For this review, take the finished solid that the model builds, in its own axes (mm). A direction names the side the tool comes from. Give positions to 0.01 mm unless a question says otherwise; leave off trailing zeros. Order: outer loops, then holes, each group sorted by start corner. A loop starts at its lowest first (then second) coordinate and runs counter-clockwise, first axis right, second up.
Item 1: Consider section A-A (x = -25.5). Give the boundary of the cut face in (y, z), plus the area to 3 significant figures.
Item 2: The part is to be moulded in two halves that separate along X. For faces 1 (the flat face through (-19.231, -31.307, 8.381)), 2 (the flat face through (-25, -21.047, 5)), 3 (the flat face through (-29.73, -31.34, 8.38)), 4 (the flat face through (-19.472, -26, 5)), say which applies: released by +X, released by -X, zero draft, split by the parting line, or undercut.
Item 3: Consider section C-C (z = 9.75). Give the boundary of the cut face in (x, y), plus the area to 3 significant figures.
Item 4: Consider section B-B (z = 15.25). Give the boundary of the cut face in (x, y), plus the area to 3 significant figures.
Item 5: For probe 1 along Y at (x, z) = (-25.5, 10); probe 2 along X at (y, z) = (-28, 1.75); probe 3 along Z at (x, y) = (-21.5, -30.25), list the stretches that pass through material, from the lowest coordinate up.
Item 6: Machinability: for faces 5 (the flat face through (-29.522, -26, 5)), 6 (the flat face through (-30.847, -26, 8)), which of the approach directions +Z, -Z, +X, -X, +Y, -Y give a long, thin tool a straight path to every point of the face, cutting with its end or side? Answer none if there is none.
```python
from build123d import *

# Parameters (mm, degrees)
F0_W     = 12.7
F0_H     = 12.7
F0_W_2   = 10.05
F0_H_2   = 10.05
F1_DEPTH = 17
F2_DEPTH = 17
F3_DEPTH = 11
F4_SIZE  = 2.2
F5_R     = 1.9


with BuildPart() as f1:
    # F0 (on Top) → F1 (new body)
    with BuildSketch(Plane.XY):
        with Locations((-24.496685, -26.072449)):
            Rectangle(F0_W, F0_H)
        with Locations((-24.496685, -26.072449)):
            Rectangle(F0_W_2, F0_H_2, mode=Mode.SUBTRACT)
    extrude(amount=F1_DEPTH)

    # F0 (on Top) → F2 (join)
    with BuildSketch(Plane.XY):
        with Locations((-24.496685, -26.072449)):
            Rectangle(F0_W_2, F0_H_2)
    extrude(amount=F2_DEPTH)

    # F0 (on Top) → F3 (cut)
    with BuildSketch(Plane.XY):
        with Locations((-24.496685, -26.072449)):
            Rectangle(F0_W_2, F0_H_2)
    extrude(amount=F3_DEPTH, mode=Mode.SUBTRACT)

    # F4
    f4_edges = [f1.edges().sort_by_distance(p)[0] for p in [
        (-18.146685, -19.722449, 8.5),
        (-30.846685, -19.722449, 8.5),
        (-30.846685, -32.422449, 8.5),
        (-18.146685, -32.422449, 8.5),
    ]]
    chamfer(f4_edges, length=F4_SIZE)

    # F5
    f5_edges = [f1.edges().sort_by_distance(p)[0] for p in [
        (-19.471685, -31.097449, 5.5),
        (-19.471685, -21.047449, 5.5),
        (-29.521685, -21.047449, 5.5),
        (-29.521685, -31.097449, 5.5),
    ]]
    fillet(f5_edges, radius=F5_R)


solid = f1.part
```
Resolved:
1. outline: (-32.42, 0) - (-31.1, 0) - (-31.1, 11) - (-21.05, 11) - (-21.05, 0) - (-19.72, 0) - (-19.72, 17) - (-32.42, 17) - close
1. area: 105 mm2
2. face 1: released by +X
2. face 2: undercut
2. face 3: released by -X
2. face 4: undercut
3. outline: (-30.85, -30.22) - (-28.65, -32.42) - (-20.35, -32.42) - (-18.15, -30.22) - (-18.15, -21.92) - (-20.35, -19.72) - (-28.65, -19.72) - (-30.85, -21.92) - close; hole (-29.52, -29.2) arc R1.9 ccw to (-27.62, -31.1) - (-21.37, -31.1) arc R1.9 ccw to (-19.47, -29.2) - (-19.47, -22.95) arc R1.9 ccw to (-21.37, -21.05) - (-27.62, -21.05) arc R1.9 ccw to (-29.52, -22.95) - close
3. area: 53.7 mm2
4. outline: (-30.85, -30.22) - (-28.65, -32.42) - (-20.35, -32.42) - (-18.15, -30.22) - (-18.15, -21.92) - (-20.35, -19.72) - (-28.65, -19.72) - (-30.85, -21.92) - close
4. area: 152 mm2
5. probe 1: y = -32.42 to -31.1, -21.05 to -19.72
5. probe 2: x = -30.85 to -29.52, -19.47 to -18.15
5. probe 3: z = 11 to 17
6. face 5: -Z
6. face 6: +Z, -Z, -X, +Y, -Y
